Check sheet for the drawn part. Datum: minimum x, y, z corner. Units: mm. Coordinates: 2 decimals unless noted, no trailing zeros. Loops run counter-clockwise (first coordinate to the right, second up) from the corner with the lowest first, then second, coordinate; pieces in that order, holes last.
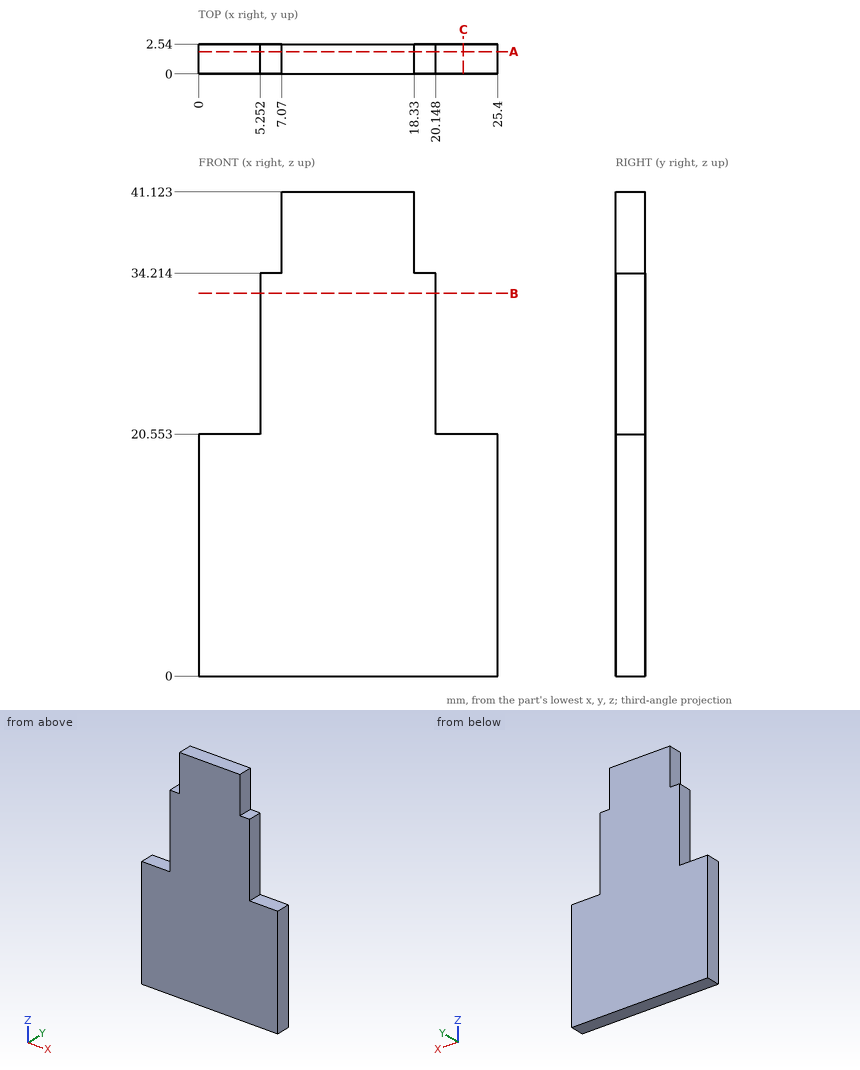
(1) Gauge pin test, flat ends, axial feed: pin 1 Ø1.5 at (x, y) = (19.5, 1) entering from +Z; pin 2 Ø1.3 at (y, z) = (1.5, 30.5) entering from +X; pin 3 Ø0.8 at (y, z) = (1.5, 36) entering from -X. Record the tip position at first contact, or that the pin passes through.
Findings:
pin 1: stops at z = 34.21
pin 2: stops at x = 20.15
pin 3: stops at x = 7.07
(2) Sectioned sample at C-C on x = 22.5. Record the cut outline in (y, z).
Findings:
outline: (0, 0) - (2.54, 0) - (2.54, 20.55) - (0, 20.55) - close
(3) Sectioned sample at A-A on y = 1.9. Record the cut outline in (x, z).
Findings:
outline: (0, 0) - (25.4, 0) - (25.4, 20.55) - (20.15, 20.55) - (20.15, 34.21) - (18.33, 34.21) - (18.33, 41.12) - (7.07, 41.12) - (7.07, 34.21) - (5.25, 34.21) - (5.25, 20.55) - (0, 20.55) - close
(4) Sectioned sample at B-B on z = 32.5. Record the cut outline in (x, y).
Findings:
outline: (5.25, 0) - (20.15, 0) - (20.15, 2.54) - (5.25, 2.54) - close
(5) Scan lines: L1, parallel to Z at x = 23.5, y = 2.15; L2, parallel to X at y = 0.85, z = 34; L3, parallel to Z at x = 20, y = 0.25. Record each from-to range of solid material in increasing order.
Findings:
L1: z = 0 to 20.55
L2: x = 5.25 to 20.15
L3: z = 0 to 34.21
